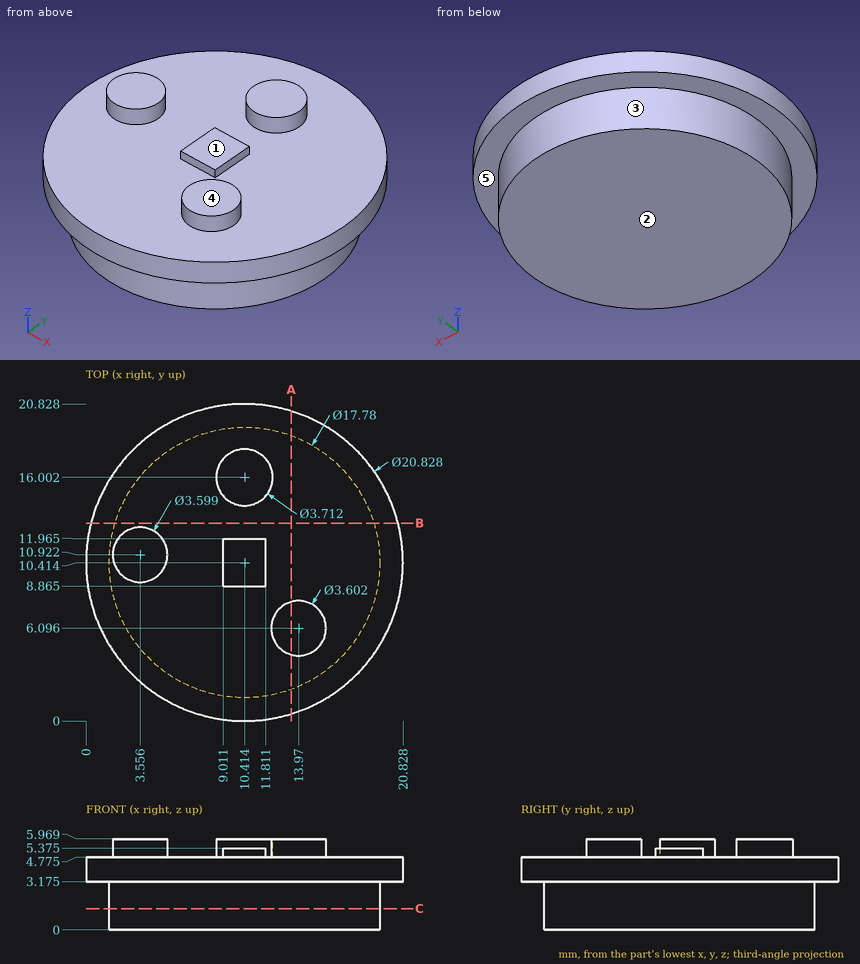
Design review of the part shown in the three views and the two pictorial views. Dimensions are in mm from the part's minimum x, y and z. A direction names the side the tool comes from. Give positions to 0.01 mm unless a question says otherwise; leave off trailing zeros. Loops run counter-clockwise (first coordinate to the right, second up) from the corner with the lowest first, then second, coordinate; pieces in that order, holes last. Notation, with made-up numbers: (23, 5) -> (62, 5) arc R7 cw to (62, 17) -> close; hole circle Ø9 at (25, 30). An arc over 180 degrees is marked (long way). Put each result on its own line as item: value. Start each with the question number.
1. Clearance check with flat-ended pins moving along their axes: P1, Ø0.7, axis at y = 11, z = 5, coming from the -X side (1 decimal); P2, Ø0.8, axis at x = 11, y = 10, coming from the +Z side (3 decimals); P3, Ø10, axis at x = 6.5, y = 2.5, coming from the +Z side (3 decimals). State where each tip first meets the part, or that it passes through.
2. For the marked faces 1 and 2, list the 3-axis set-ups (+Z, -Z, +X, -X, +Y, -Y) from which the entire face can be reached by the end or side of a thin tool; tool diameter is ignored.
3. We need section C-C on z = 1.4. State the section outline as (x, y) points, then the cut area to 3 significant figures.
4. We need section B-B on y = 13. State the section outline as (x, z) points (1 decimal).
5. Mouldability with a two-part tool opening along Z and no side actions: class the marked faces 3, 4 and 5 as released by +Z, released by -Z, zero draft, split by the parting line, or undercut.
6. We need section A-A on x = 13.5. State the section outline as (y, z) points (1 decimal).
7. Wall thickness on probe 1 along Z at (x, y) = (16.75, 11.5) (1 decimal); probe 2 along Z at (x, y) = (3.5, 3) (1 decimal); probe 3 along Y at (x, z) = (2.5, 5.6) (1 decimal): over which ranges is each line inside the solid? List them lowest first.
Determined:
1. P1: x = 0
1. P2: z = 5.375
1. P3: z = 4.775
2. face 1: +Z, +X, -Y
2. face 2: -Z, +X, -X, +Y, -Y
3. outline: circle Ø17.78 at (10.41, 10.41)
3. area: 248 mm^2
4. outline: (0.3, 3.2) -> (1.9, 3.2) -> (1.9, 0) -> (18.9, 0) -> (18.9, 3.2) -> (20.5, 3.2) -> (20.5, 4.8) -> (0.3, 4.8) -> close
5. face 3: zero draft
5. face 4: released by +Z
5. face 5: released by -Z
6. outline: (0.5, 3.2) -> (2.1, 3.2) -> (2.1, 0) -> (18.8, 0) -> (18.8, 3.2) -> (20.4, 3.2) -> (20.4, 4.8) -> (7.8, 4.8) -> (7.8, 6) -> (4.4, 6) -> (4.4, 4.8) -> (0.5, 4.8) -> close
7. probe 1: 0 to 4.8
7. probe 2: 3.2 to 4.8
7. probe 3: 9.5 to 12.4
